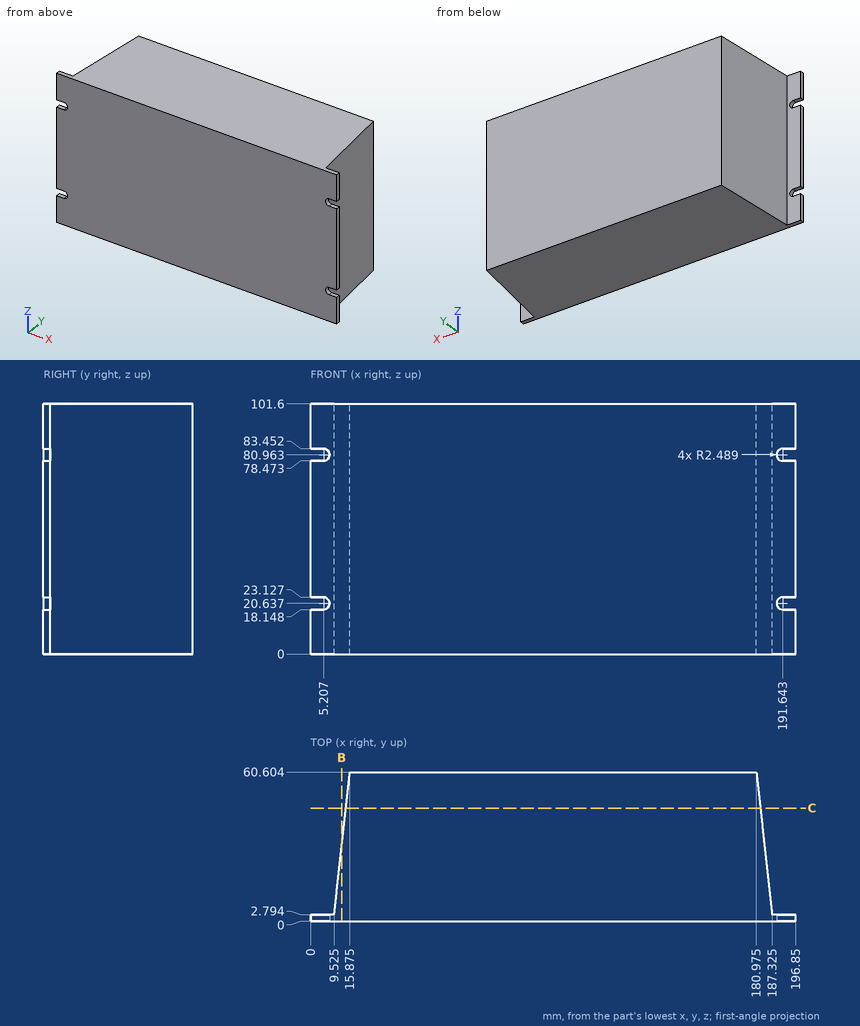
Here's the drawing with two shaded views (mm, measured from the low corner). I have some questions. Round coordinates to 2 decimals unless told otherwise and drop trailing zeros. Order: outer loops, then holes, each group sorted by start corner. A loop starts at its lowest first (then second) coordinate and runs counter-clockwise, first axis right, second up. Notation, with made-up numbers: M 60.5,53 L 105.5,53 A19 cw 105.5,68 Z; hole C 6.5,58.25 d4. An arc over 180 degrees is marked long. Answer in a Markdown table with one row per item.
Item 1: Imagine slicing it at C-C, the plane y = 46. Write out the boundary of the cut face in (x, z), and give its area (3 significant figures).
A:
| item | result |
|---|---|
| outline | M 14.27,0 L 182.58,0 L 182.58,101.6 L 14.27,101.6 Z |
| area | 17,100 mm2 |
Item 2: Imagine slicing it at B-B, the plane x = 12.5. Write out the boundary of the cut face in (y, z).
A:
| item | result |
|---|---|
| outline | M 0,0 L 29.88,0 L 29.88,101.6 L 0,101.6 Z |
Item 3: If I drill on L1, parallel to X at y = 29, z = 7.5; L2, parallel to X at y = 45, z = 18, over which ranges is the centre line in solid material (lowest first)? Write a range as from..to.
A:
| item | result |
|---|---|
| L1 | x = 12.4..184.45 |
| L2 | x = 14.16..182.69 |
Item 4: I'm going to push flat-ended pins straight in: pin 1 (5 mm diameter, centred on x = 5, z = 44.5, fed in from +Y); pin 2 (2 mm diameter, centred on y = 40, z = 30, fed in from +X); pin 3 (2 mm diameter, centred on y = 22.5, z = 77, fed in from -X). Where does each tip first touch, or does it pass through?
A:
| item | result |
|---|---|
| pin 1 | stops at y = 2.79 |
| pin 2 | stops at x = 183.35 |
| pin 3 | stops at x = 11.58 |
